Can you work these out from the model? Positions are in its coordinate system, mm. A direction names the side the tool comes from. Give positions to 0.01 mm unless a question says otherwise; leave off trailing zeros. Loops run counter-clockwise (first coordinate to the right, second up) from the corner with the lowest first, then second, coordinate; pieces in that order, holes last. Notation, with made-up numbers: (83, 15.5) -> (100, 15.5) arc R12 ccw to (100, 38.5) -> close; hole circle Ø8 at (29, 42.25). An arc over 180 degrees is marked (long way). Use CSV: the item, a comma, the result in double quotes.
Autodesk Inventor part; units mm, degrees
ref_plane "YZ Plane" through (0, 0, 0) normal (1, 0, 0) x (0, 1, 0)
ref_plane "XZ Plane" through (0, 0, 0) normal (0, 1, 0) x (-1, 0, 0)
ref_plane "XY Plane" through (0, 0, 0) normal (0, 0, 1) x (1, 0, 0)
sketch "Sketch1" plane through (0, 0, 0) normal (0, 1, 0) x (-1, 0, 0)
  line L0 (28, 33) -> (-28, 33)
  line L1 (-33, 28) -> (-33, -28)
  line L2 (-28, -33) -> (28, -33)
  line L3 (33, -28) -> (33, 28)
  line L4 (33, 33) -> (-33, -33) construction
  line L5 (-33, 33) -> (33, -33) construction
  arc A0 (28, -33) -> (33, -28) centre (28, -28) ccw
  arc A1 (33, 28) -> (28, 33) centre (28, 28) ccw
  arc A2 (-28, 33) -> (-33, 28) centre (-28, 28) ccw
  arc A3 (-33, -28) -> (-28, -33) centre (-28, -28) ccw
  point P0 (0, 0)
  dimension "d0" = 66
  dimension "d1" = 66
  dimension "d4" = 5
extrude "Extrusion1" add sketch "Sketch1" along normal blind 35
sketch "Sketch2" plane through (0, 35, 0) normal (0, 1, 0) x (1, 0, 0)
  line L0 (0, 0) -> (-10, 0)
  line L1 (0, 0) -> (0, -10)
  circle A0 centre (26, 26) radius 5.35
  circle A1 centre (0, 26) radius 5.35
  circle A2 centre (-26, 26) radius 5.35
  circle A3 centre (26, 0) radius 5.35
  circle A4 centre (0, 0) radius 5.35
  circle A5 centre (-26, 0) radius 5.35
  circle A6 centre (26, -26) radius 5.35
  circle A7 centre (0, -26) radius 5.35
  circle A8 centre (-26, -26) radius 5.35
  dimension "d8" = 10
  dimension "d9" = 10
  dimension "d10" = 10.7
  dimension "d11" = 26
  dimension "d12" = 26
  dimension "d15" = 26
  dimension "d18" = 26
extrude "Extrusion2" cut sketch "Sketch2" against normal blind 35 contours A0 | A1 | A2 | A3 | A5 | A6 | A7 | A8
sketch "Sketch4" plane through (0, 0, 0) normal (0, -1, 0) x (1, 0, 0)
  line L0 (37.5, 37.5) -> (-37.5, -37.5) construction
  line L1 (-37.5, 37.5) -> (37.5, -37.5) construction
  line L2 (-41, -38) -> (-41, 38)
  line L3 (41, -41) -> (-41, 41) construction
  line L4 (-41, -41) -> (41, 41) construction
  circle A0 centre (-37.5, 37.5) radius 1.85
  line L5 (38, 41) -> (-38, 41)
  line L6 (-38, -41) -> (38, -41)
  line L7 (41, -38) -> (41, 38)
  line L8 (41, 41) -> (-41, -41) construction
  line L9 (-41, 41) -> (41, -41) construction
  circle A1 centre (-37.5, -37.5) radius 1.85
  circle A2 centre (37.5, 37.5) radius 1.85
  circle A3 centre (37.5, -37.5) radius 1.85
  line L10 (-41, -38) -> (-41, -41)
  line L11 (-38, -41) -> (-41, -41)
  line L12 (-41, 38) -> (-41, 41)
  line L13 (-38, 41) -> (-41, 41)
  line L14 (38, 41) -> (41, 41)
  line L15 (41, 38) -> (41, 41)
  line L16 (41, -38) -> (41, -41)
  line L17 (41, -41) -> (38, -41)
  point P0 (0, 0)
  dimension "d28" = 75
  dimension "d29" = 75
  dimension "d31" = 82
  dimension "d56" = 3.7
  dimension "d68" = 75
  dimension "d71" = 75
extrude "Extrusion4" add sketch "Sketch4" along normal blind 3
thread "Thread5"
thread "Thread6"
thread "Thread7"
thread "Thread8"
properties part number "Aluminium Container 0805" material "Aluminum 6061"
(1) If we section it at C-C, the plane y = 19.5: Give the number of separate pieces and of enclosed holes in the cut face, then the cut area to 3 significant figures.
Answer sheet:
separate pieces,"1"
enclosed holes,"8"
area,"3,620 mm2"
(2) We'd pull the mould along X, two halves only. Please class faces 4 (the face through (31, 17, -32)), 5 (the face through (-31, 17, 32)), 6 (the face through (36.032, -1.479, -36.374)): released by +X, released by -X, zero draft, split by the parting line, or undercut.
Answer sheet:
face 4,"released by +X"
face 5,"released by -X"
face 6,"undercut"
(3) Will these pins go through, and if not, where does the flat tip stop? pin 1 Ø8 at (y, z) = (5.5, -8.5) entering from -X; pin 2 Ø8 at (x, y) = (10.5, 18) entering from -Z; pin 3 Ø5.5 at (x, z) = (-27, -27.5) entering from +Y.
Answer sheet:
pin 1,"stops at x = -33"
pin 2,"stops at z = -33"
pin 3,"stops at y = 0"
(4) If we section it at D-D, the plane z = 0: Write out the boundary of the cut face in (x, y).
Answer sheet:
outline,"(-41, -3) -> (41, -3) -> (41, 0) -> (33, 0) -> (33, 35) -> (31.35, 35) -> (31.35, 0) -> (20.65, 0) -> (20.65, 35) -> (-20.65, 35) -> (-20.65, 0) -> (-31.35, 0) -> (-31.35, 35) -> (-33, 35) -> (-33, 0) -> (-41, 0) -> close"
(5) Which directions (+Z, -Z, +X, -X, +Y, -Y) give clear straight access to the entire face, cutting with the end or side of a thin tool? Please do faces 1 (the face through (21.754, 17.745, 3.255)), 2 (the face through (0, 17, -33)), 3 (the face through (32, 17, 31)).
Answer sheet:
face 1,"+Y"
face 2,"-Z, +X, -X, +Y"
face 3,"+Z, +X, +Y"
(6) If I drill on L1, parallel to Z at x = 37.5, y = -0.7; L2, parallel to X at y = 12, z = -26; L3, parallel to X at y = 24, z = 0, over which ranges is the centre line in solid material (lowest first)? Write a range as from..to.
Answer sheet:
L1,"z = -41..-39.35, -35.65..35.65, 39.35..41"
L2,"x = -33..-31.35, -20.65..-5.35, 5.35..20.65, 31.35..33"
L3,"x = -33..-31.35, -20.65..20.65, 31.35..33"
(7) If we section it at A-A, the plane x = 37.5: Write out the boundary of the cut face in (y, z).
Answer sheet:
outline,"(-3, -41) -> (0, -41) -> (0, -39.35) -> (-3, -39.35) -> close; (-3, -35.65) -> (0, -35.65) -> (0, 35.65) -> (-3, 35.65) -> close; (-3, 39.35) -> (0, 39.35) -> (0, 41) -> (-3, 41) -> close"
(8) If we section it at B-B, the plane z = -37.5: Write out the boundary of the cut face in (x, y), then the cut area to 3 significant figures.
Answer sheet:
outline,"(-41, -3) -> (-39.35, -3) -> (-39.35, 0) -> (-41, 0) -> close; (-35.65, -3) -> (35.65, -3) -> (35.65, 0) -> (-35.65, 0) -> close; (39.35, -3) -> (41, -3) -> (41, 0) -> (39.35, 0) -> close"
area,"224 mm2"
